Source: three-view drawing plus pictorial views. Frame: mm from the lowest corner of the part. A direction names the side the tool comes from. Give positions to 0.01 mm unless a question says otherwise; leave off trailing zeros. Order: outer loops, then holes, each group sorted by start corner. A loop starts at its lowest first (then second) coordinate and runs counter-clockwise, first axis right, second up.
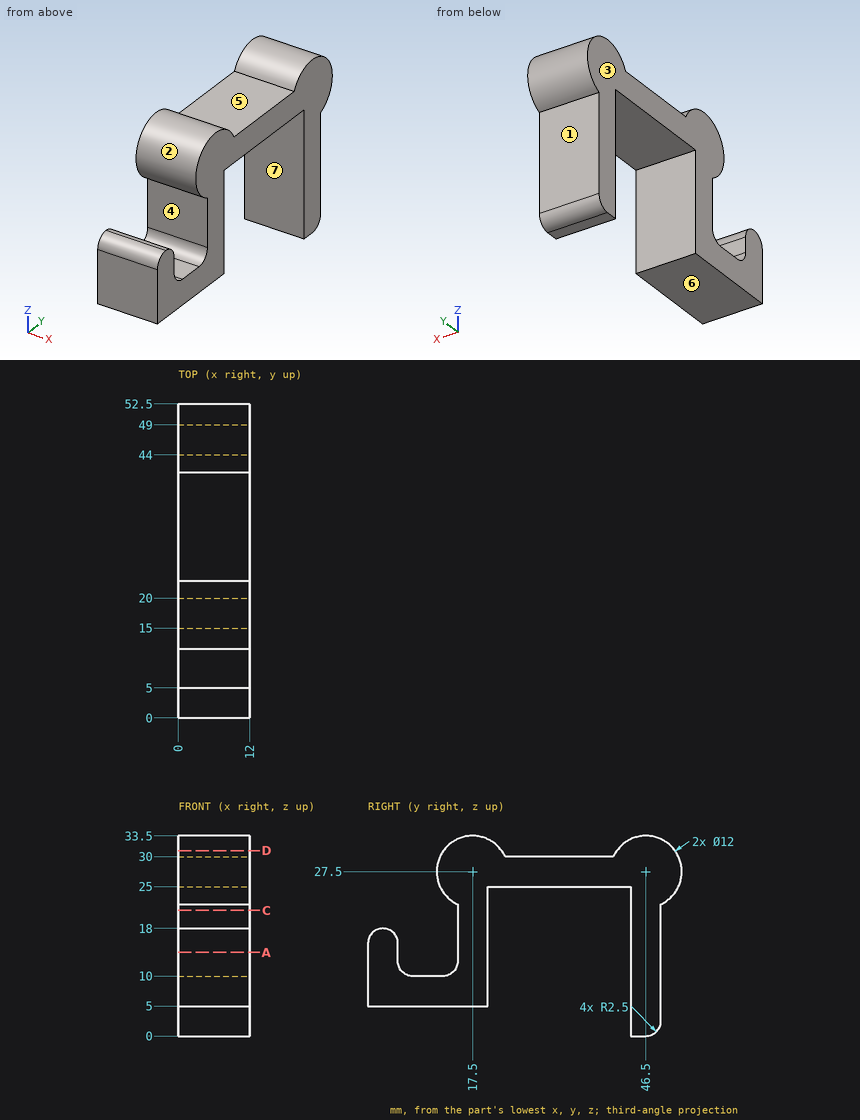
(1) Section D-D, the plane z = 31. Return loops of the section in (x, y).
(2) Access query for the marked faces 4, 5, 6 and 7. Directions: +Z, -Z, +X, -X, +Y, -Y. A direction counts if a zero-diameter tool reaches every point of the face in a straight line with its end or side. Return the directions, or none.
(3) Section A-A, the plane z = 14. Return loops of the section in (x, y).
(4) Draft query along Y for the marked faces 1, 2 and 3. Return one class per face: +Y half, -Y half, draft (parallel to the pull), parting line (faces both ways), or undercut.
(5) Pin query (flat end, axial travel): pin 1 Ø1.5 at (x, z) = (6, 13.5) entering from +Y; pin 2 Ø3 at (x, y) = (9.5, 31) entering from +Z; pin 3 Ø1 at (x, y) = (9, 28) entering from -Z; pin 4 Ø1 at (x, z) = (7.5, 5) entering from -Y. Return the tip coordinate at first contact, or that it passes through.
(6) Section C-C, the plane z = 21. Return loops of the section in (x, y).
(7) Line query: line 1 along Y through (x, z) = (8, 15); line 2 along Y through (x, z) = (1, 20); line 3 along Z through (x, y) = (2, 37). Output: solid intervals per line, ascending.
Checks:
1. outline: (0, 12.63) - (12, 12.63) - (12, 22.37) - (0, 22.37) - close; (0, 41.63) - (12, 41.63) - (12, 51.37) - (0, 51.37) - close
2. face 4: +X, -X
2. face 5: +Z, +X, -X
2. face 6: -Z, +X, -X, -Y
2. face 7: -Z, +X, -X
3. outline: (0, 0) - (12, 0) - (12, 5) - (0, 5) - close; (0, 15) - (12, 15) - (12, 20) - (0, 20) - close; (0, 44) - (12, 44) - (12, 49) - (0, 49) - close
4. face 1: +Y half
4. face 2: undercut
4. face 3: draft
5. pin 1: stops at y = 49
5. pin 2: stops at z = 30
5. pin 3: stops at z = 25
5. pin 4: stops at y = 0
6. outline: (0, 15) - (12, 15) - (12, 20) - (0, 20) - close; (0, 44) - (12, 44) - (12, 49) - (0, 49) - close
7. line 1: y = 0 to 5, 15 to 20, 44 to 49
7. line 2: y = 15 to 20, 44 to 49
7. line 3: z = 25 to 30
